from build123d import *

# Parameters (mm, degrees)
SKETCH1_W               = 254
SKETCH1_H               = 254
BOSS_EXTRUDE1_DEPTH     = 6.35
CAVITY1_START           = -6.35
CAVITY1_OUTLINE_R       = 12.7
CAVITY1_DEPTH           = 12.7
CUT_EXTRUDE2_DEPTH      = 285.051619429
CUT_EXTRUDE2_DEPTH_BACK = 285.051619429
SKETCH3_W               = 127
SKETCH3_H               = 12.7
MOVE_FACE_SLOT_BY       = 0.762
MOVE_FACE_SLOT_2_BY     = 0.762
MOVE_FACE_SLOT_3_BY     = 0.762
FILLET1_R               = 3.175
MOVE_FACE_HOLE_BY       = 0.635


# Read off the part's stored shape, not the designer's step: Cavity1
with BuildPart() as part:
    # Sketch1 → Boss-Extrude1 (new, symmetric)
    with BuildSketch(Plane(origin=(0, 0, 0), x_dir=(1, 0, 0), z_dir=(0, 1, 0))):
        with Locations((0, 127)):
            Rectangle(SKETCH1_W, SKETCH1_H)
    extrude(amount=BOSS_EXTRUDE1_DEPTH, both=True)

    # Cavity1 outline → Cavity1 (cut)
    with BuildSketch(Plane(origin=(0, 0, 0), x_dir=(1, 0, 0), z_dir=(0, 1, 0)).offset(CAVITY1_START)):
        with Locations((-85.75, 190.5)):
            Circle(CAVITY1_OUTLINE_R)
    extrude(amount=CAVITY1_DEPTH, mode=Mode.SUBTRACT)

    # Sketch3 → Cut-Extrude2 (cut, two sides: drawn at the far end of the back side and taken through both)
    with BuildSketch(Plane(origin=(0, 0, 0), x_dir=(1, 0, 0), z_dir=(0, 1, 0)).offset(-CUT_EXTRUDE2_DEPTH_BACK)):
        with Locations((-63.5, 57.15)):
            Rectangle(SKETCH3_W, SKETCH3_H)
    extrude(amount=CUT_EXTRUDE2_DEPTH + CUT_EXTRUDE2_DEPTH_BACK, mode=Mode.SUBTRACT)

    # Move Face slot: a face moved inward by 0.762
    extrude(part.faces().sort_by_distance((0, 0, -57.15))[0], amount=MOVE_FACE_SLOT_BY, dir=(1, 0, 0), mode=Mode.SUBTRACT)

    # Move Face slot 2: a face moved inward by 0.762
    extrude(part.faces().sort_by_distance((-63.5, 0, -63.5))[0], amount=MOVE_FACE_SLOT_2_BY, dir=(0, 0, -1), mode=Mode.SUBTRACT)

    # Move Face slot 3: a face moved inward by 0.762
    extrude(part.faces().sort_by_distance((-63.5, 0, -50.8))[0], amount=MOVE_FACE_SLOT_3_BY, dir=(0, 0, 1), mode=Mode.SUBTRACT)

    # Fillet1
    fillet1_edges = [part.edges().sort_by_distance(p)[0] for p in [
        (-127, 0, -50.038),
        (-127, 0, -64.262),
        (0.762, 0, -64.262),
        (0.762, 0, -50.038),
    ]]
    fillet(fillet1_edges, radius=FILLET1_R)

    # Move Face hole: a curved face moved inward by 0.635
    add(Solid.thicken(part.faces().sort_by_distance((-98.45, 0, -190.5))[0], -MOVE_FACE_HOLE_BY), mode=Mode.SUBTRACT)


solid = part.part
CAD build for the part. Positions are in the model's coordinates, mm. A direction names the side the tool comes from. Coordinates: 2 decimals unless noted, no trailing zeros. Order: outer loops, then holes, each group sorted by start corner. A loop starts at its lowest first (then second) coordinate and runs counter-clockwise, first axis right, second up. Notation, with made-up numbers: (32.25, 69.5) -> (68.25, 69.5) arc R24 cw to (68.25, 100.5) -> close; hole circle Ø10 at (72.5, -19). An arc over 180 degrees is marked (long way). Answer in a Markdown table with one row per item.
1) Band-saw the part on A-A (x = -85.75). List the corners of the cut face in (y, z) (3 decimals).
Check values:
| item | result |
|---|---|
| outline | (-6.35, -254) -> (6.35, -254) -> (6.35, -203.835) -> (-6.35, -203.835) -> close; (-6.35, -177.165) -> (6.35, -177.165) -> (6.35, -64.262) -> (-6.35, -64.262) -> close; (-6.35, -50.038) -> (6.35, -50.038) -> (6.35, 0) -> (-6.35, 0) -> close |
2) Band-saw the part on C-C (y = 2.5). List the corners of the cut face in (x, z) (3 decimals), and give its area (3 significant figures).
Check values:
| item | result |
|---|---|
| outline | (-127, -254) -> (127, -254) -> (127, 0) -> (-127, 0) -> (-127, -46.863) arc R3.175 ccw to (-123.825, -50.038) -> (-2.413, -50.038) arc R3.175 cw to (0.762, -53.213) -> (0.762, -61.087) arc R3.175 cw to (-2.413, -64.262) -> (-123.825, -64.262) arc R3.175 ccw to (-127, -67.437) -> close; hole circle Ø26.67 at (-85.75, -190.5) |
| area | 62,100 mm2 |
3) Flat gauge pins, fed straight in: P1, Ø16, axis at x = -85.75, z = -190.5, coming from the +Y side; P2, Ø2.5, axis at y = -0.5, z = -56.5, coming from the -X side. Where does each tip first touch, or does it go through?
Check values:
| item | result |
|---|---|
| P1 | through |
| P2 | x = 0.76 |
4) Mould opens along Z. For faces 1 (the face through (0.762, 0, -57)), 2 (the face through (-2, 0, -254)), 3 (the face through (127, 0, -125)) say: pulls with the +Z half, pulls with the -Z half, needs draft (parallel to the pull), parting line crosses it, or undercut.
Check values:
| item | result |
|---|---|
| face 1 | undercut |
| face 2 | pulls with the -Z half |
| face 3 | needs draft |
5) Drill centre lines: line 1 (Z direction, x = -85.75, y = 0.75) (3 decimals); line 2 (X direction, y = 0, z = -190.5) (3 decimals); line 3 (Z direction, x = -10.5, y = 2.5). Where is each one in solid material? Low to high.
Check values:
| item | result |
|---|---|
| line 1 | -254 to -203.835, -177.165 to -64.262, -50.038 to 0 |
| line 2 | -127 to -99.085, -72.415 to 127 |
| line 3 | -254 to -64.26, -50.04 to 0 |
6) Band-saw the part on B-B (z = -190.5). List the corners of the cut face in (x, y) (3 decimals).
Check values:
| item | result |
|---|---|
| outline | (-127, -6.35) -> (-99.085, -6.35) -> (-99.085, 6.35) -> (-127, 6.35) -> close; (-72.415, -6.35) -> (127, -6.35) -> (127, 6.35) -> (-72.415, 6.35) -> close |
7) Which spindle directions (+Z, -Z, +X, -X, +Y, -Y) get a long thin tool onto all of the face, cutting with end or side? Do faces 4 (the face through (-95.58, -0.09, -199.51)), 5 (the face through (-64, 0, -50.038)). Say none if no direction does.
Check values:
| item | result |
|---|---|
| face 4 | +Y, -Y |
| face 5 | -X, +Y, -Y |
